Geometry check sheet. Reference: the model listing, model coordinates, mm. A direction names the side the tool comes from. Give positions to 0.01 mm unless a question says otherwise; leave off trailing zeros. Loops run counter-clockwise (first coordinate to the right, second up) from the corner with the lowest first, then second, coordinate; pieces in that order, holes last. Notation, with made-up numbers: (-6, 4) -> (31, 4) arc R19 ccw to (31, 10) -> close; hole circle Ø9 at (-26, 38.25). An arc over 180 degrees is marked (long way). Answer in a Markdown table with one row per item. Add a question column.
```python
from build123d import *

# Parameters (mm, degrees)
BOSS_EXTRUDE1_DEPTH = 0.94
CIRPATTERN1_COUNT   = 3


with BuildPart() as part:
    # Sketch2 → Revolve1 (revolve)
    with BuildSketch(Plane(origin=(0, 0, 0), x_dir=(0, 0, -1), z_dir=(1, 0, 0))):
        with BuildLine():
            Line((-1, 17), (1, 17))
            ThreePointArc((1, 17), (3.49313133, 8.661985943), (4.334666688, 0))
            Line((4.334666688, 0), (-4.455333312, 0))
            ThreePointArc((-4.455333312, 0), (-3.58275786, 8.673801478), (-1, 17))
        make_face()
    revolve(axis=Axis((0, 0, 0), (0, 0, -1)))

    # Sketch3 → Boss-Extrude1 (add, symmetric)
    with BuildSketch(Plane.XY):
        with BuildLine():
            Line((-5.15, 16.201157366), (-5.15, 17.52))
            ThreePointArc((-5.15, 17.52), (-4.335756852, 19.485756852), (-2.37, 20.3))
            Line((-2.37, 20.3), (2.37, 20.3))
            ThreePointArc((2.37, 20.3), (4.335756852, 19.485756852), (5.15, 17.52))
            Line((5.15, 17.52), (5.15, 16.201157366))
            ThreePointArc((5.15, 16.201157366), (0, 17), (-5.15, 16.201157366))
        make_face()
    boss_extrude1 = extrude(amount=BOSS_EXTRUDE1_DEPTH, both=True)

    # CirPattern1: Boss-Extrude1 ×3 about axis
    cirpattern1_axis = Axis((0, 0, 0), (0, 0, 1))
    for i in range(1, CIRPATTERN1_COUNT):
        add(boss_extrude1.rotate(cirpattern1_axis, i * 360 / CIRPATTERN1_COUNT))


solid = part.part
```
1. Release check for a two-part mould opening along Y. For faces 1 (the face through (-12.019, -12.886, 0.013)), 2 (the face through (-17.18, -3.97, 0.01)), 3 (the face through (19.035, -5.959, 0.013)), 4 (the face through (-16, -9, -0.94)) record: released by +Y, released by -Y, zero draft, split by the parting line, or undercut.
2. Sectioned sample at B-B (y = -15). Enter the section's corners in (x, z), plus the area to 3 significant figures.
3. Sectioned sample at D-D (x = -14.5). Enter the section's corners in (y, z), plus the area to 3 significant figures.
4. Sectioned sample at A-A (x = 0). Enter the section's corners in (y, z), plus the area to 3 significant figures.
5. Material ranges on L1, parallel to X at y = 0.5, z = 0; L2, parallel to Z at x = -6.5, y = 12.5; L3, parallel to Z at x = 11.5, y = 12, recorded low to high. Write a range as from..to.
6. Gauge pin test, flat ends, axial feed: pin 1 Ø1.1 at (y, z) = (17, 0) entering from -X; pin 2 Ø1.5 at (x, y) = (-6, 8) entering from -Z; pin 3 Ø4.5 at (x, y) = (1.5, 19) entering from +Z. Record the tip position at first contact, or that the pin passes through.
7. Access from +Z, -Z, +X, -X, +Y, -Y to the whole of each face (thin tool, end or side, straight path). Record for faces 5 (the face through (5.15, 17, 0)), 6 (the face through (-16, -9, 0.94)), 7 (the face through (-5.15, 17, 0)).
Response:
| question | item | result |
|---|---|---|
| 1 | face 1 | released by -Y |
| 1 | face 2 | undercut |
| 1 | face 3 | split by the parting line |
| 1 | face 4 | zero draft |
| 2 | outline | (-8, -1) arc R42.43 ccw to (8, -1) -> (8, 1) arc R40.88 ccw to (-8, 1) -> close |
| 2 | area | 48.6 mm2 |
| 3 | outline | (-13.54, -0.94) -> (-8.87, -0.94) -> (-8.87, -1) arc R42.6 ccw to (8.87, -1) -> (8.87, 1) arc R41.06 ccw to (-8.87, 1) -> (-8.87, 0.94) -> (-13.54, 0.94) -> close |
| 3 | area | 66.9 mm2 |
| 4 | outline | (-17, -1) arc R45 ccw to (17, -1) -> (17, -0.94) -> (20.3, -0.94) -> (20.3, 0.94) -> (17, 0.94) -> (17, 1) arc R43.55 ccw to (-17, 1) -> close |
| 4 | area | 229 mm2 |
| 5 | L1 | x = -16.99..16.99 |
| 5 | L2 | z = -2.07..2.11 |
| 5 | L3 | z = -1.15..1.16 |
| 6 | pin 1 | stops at x = -5.15 |
| 6 | pin 2 | stops at z = -3.37 |
| 6 | pin 3 | stops at z = 1.08 |
| 7 | face 5 | +Z, -Z, +X, +Y |
| 7 | face 6 | +Z, -X, -Y |
| 7 | face 7 | +Z, -Z, -X, +Y |
